Model file for the job. Use its own axes, mm. A direction names the side the tool comes from. Round coordinates to 2 decimals unless told otherwise and drop trailing zeros. Order: outer loops, then holes, each group sorted by start corner. A loop starts at its lowest first (then second) coordinate and runs counter-clockwise, first axis right, second up. Notation, with made-up numbers: (-24, 22.25) - (27, 22.25) arc R19 ccw to (27, 58.25) - close; hole circle Ø9 at (-9.5, -22.75). An arc over 180 degrees is marked (long way). Answer as CSV lines item,"result". Start each with the question number.
1. Band-saw the part on A-A on y = 193. List the corners of the cut face in (x, z) (3 decimals).
2. Band-saw the part on B-B on x = 8.75. List the corners of the cut face in (y, z) (3 decimals).
3. 3-axis set-ups, long thin cutter, end or side, ignore diameter. For faces 1 (the face through (10, 169, -3.175)), 2 (the face through (8, 169, -12.7)), 3 (the face through (3.175, 169, -9)): which of +Z, -Z, +X, -X, +Y, -Y reach the whole face in a straight line?
4. Pin check, flat tips, straight feed: pin 1 Ø0.8 at (x, y) = (1.5, 114.5) entering from -Z; pin 2 Ø1.3 at (y, z) = (216, -2) entering from +X; pin 3 Ø6 at (y, z) = (143.5, -3) entering from -X. Stop position of each tip, or through.
5. Wall check: line 1 along Z through (x, y) = (11.25, 24) (3 decimals); line 2 along X through (y, z) = (199.5, -7) (3 decimals); line 3 along Z through (x, y) = (6, 272). Give the ranges that are in metal, low to high. Write a range as [from, to].
```python
from build123d import *

# Parameters (mm, degrees)
BOSS_EXTRUDE1_DEPTH = 342.9


with BuildPart() as part:
    # Sketch1 → Boss-Extrude1 (new body)
    with BuildSketch(Plane(origin=(0, 0, 0), x_dir=(1, 0, 0), z_dir=(0, 1, 0))):
        with BuildLine():
            Line((3.175, 12.7), (12.7, 12.7))
            Line((12.7, 12.7), (12.7, 3.175))
            Line((12.7, 3.175), (6.35, 3.175))
            Line((6.35, 3.175), (6.35, 0.508))
            ThreePointArc((6.35, 0.508), (2.349005221, 2.349005221), (0.508, 6.35))
            Line((0.508, 6.35), (3.175, 6.35))
            Line((3.175, 6.35), (3.175, 12.7))
        make_face()
    extrude(amount=BOSS_EXTRUDE1_DEPTH)


solid = part.part
```
Reply:
1,outline,"(0.508, -6.35) - (3.175, -6.35) - (3.175, -12.7) - (12.7, -12.7) - (12.7, -3.175) - (6.35, -3.175) - (6.35, -0.508) arc R6.35 ccw to start"
2,outline,"(0, -12.7) - (342.9, -12.7) - (342.9, -3.175) - (0, -3.175) - close"
3,face 1,"+Z, +X, +Y, -Y"
3,face 2,"-Z, +X, -X, +Y, -Y"
3,face 3,"-Z, -X, +Y, -Y"
4,pin 1,"stops at z = -6.35"
4,pin 2,"stops at x = 6.35"
4,pin 3,"stops at x = 0.54"
5,line 1,"z = [-12.7, -3.175]"
5,line 2,"x = [3.175, 12.7]"
5,line 3,"z = [-12.7, -0.54]"
